Could you check a few things on this model? Use its own coordinates, in mm. Face numbers are marked on the shaded views. A direction names the side the tool comes from. Give positions to 0.01 mm unless a question says otherwise; leave off trailing zeros. Order: outer loops, then holes, each group sorted by start corner. A loop starts at its lowest first (then second) coordinate and runs counter-clockwise, first axis right, second up. Notation, with made-up numbers: (79.25, -35) -> (137.25, -35) arc R26 cw to (137.25, 0) -> close; hole circle Ø3 at (-10, -40). An arc over 180 degrees is marked (long way). One line per item, written item: value.
```python
from build123d import *
from build123d.topology import SkipClean

# Parameters (mm, degrees)
BOSS_EXTRUDE1_DEPTH          = 13.3
CHAMFER1_SIZE                = 2
CIRPATTERN1_COUNT            = 6
CHAMFER1_OF_CIRPATTERN1_SIZE = 2
CHAMFER2_SIZE                = 2
FILLET1_R                    = 1


with BuildPart() as part:
    # Sketch1 → Revolve1 (revolve)
    with BuildSketch(Plane.XY, mode=Mode.PRIVATE) as revolve1_sk:
        Polygon((-16.5, 0), (-29, 0), (-29, -8), (-23.5, -8), (-23.5, -13), (-26.75, -13), (-26.75, -17), (-20.5, -17), (-20.5, -19), (-15.5, -19), (-15.5, -6.5), (-16.5, -6.5), align=None)
    revolve(revolve1_sk.sketch.rotate(Axis((0, 0, 0), (0, -1, 0)), 270), axis=Axis((0, 0, 0), (0, -1, 0)))

    # Sketch2 → Boss-Extrude1 (add)
    with SkipClean():  # the faces are left unmerged after this step: merging them gives an invalid solid
        with BuildSketch(Plane(origin=(0, 0, 0), x_dir=(1, 0, 0), z_dir=(0, 1, 0))):
            with BuildLine():
                Line((5.154427, 16.199749), (8.792846, 27.634867))
                ThreePointArc((8.792846, 27.634867), (0, 29), (-8.792846, 27.634867))
                Line((-8.792846, 27.634867), (-5.154427, 16.199749))
                ThreePointArc((-5.154427, 16.199749), (0, 17), (5.154427, 16.199749))
            make_face()
        boss_extrude1 = extrude(amount=BOSS_EXTRUDE1_DEPTH)

    # Chamfer1
    chamfer1_edges = [part.edges().sort_by_distance(p)[0] for p in [
        (6.973637, 13.3, -21.917308),
        (-6.973637, 13.3, -21.917308),
    ]]
    chamfer(chamfer1_edges, length=CHAMFER1_SIZE)

    # CirPattern1: Boss-Extrude1 ×6 about axis
    with SkipClean():  # the faces are left unmerged after this step: merging them gives an invalid solid
        cirpattern1_axis = Axis((0, 0, 0), (0, 1, 0))
        for i in range(1, CIRPATTERN1_COUNT):
            add(boss_extrude1.rotate(cirpattern1_axis, i * 360 / CIRPATTERN1_COUNT))

    # Chamfer1 of CirPattern1
    chamfer1_of_cirpattern1_edges = [part.edges().sort_by_distance(p)[0] for p in [
        (-15.494127, 13.3, -16.998),
        (-22.467764, 13.3, -4.919308),
        (-22.467764, 13.3, 4.919308),
        (-15.494127, 13.3, 16.998),
        (-6.973637, 13.3, 21.917308),
        (6.973637, 13.3, 21.917308),
        (15.494127, 13.3, 16.998),
        (22.467764, 13.3, 4.919308),
        (22.467764, 13.3, -4.919308),
        (15.494127, 13.3, -16.998),
    ]]
    chamfer(chamfer1_of_cirpattern1_edges, length=CHAMFER1_OF_CIRPATTERN1_SIZE)

    # Chamfer2
    chamfer2_edges = [part.edges().sort_by_distance(p)[0] for p in [
        (0, -17, -26.75),
        (0, -8, -29),
    ]]
    chamfer(chamfer2_edges, length=CHAMFER2_SIZE)

    # Fillet1
    fillet1_edges = [part.edges().sort_by_distance(p)[0] for p in [
        (0, -13, -23.5),
        (0, -8, -23.5),
    ]]
    fillet(fillet1_edges, radius=FILLET1_R)


solid = part.part
```
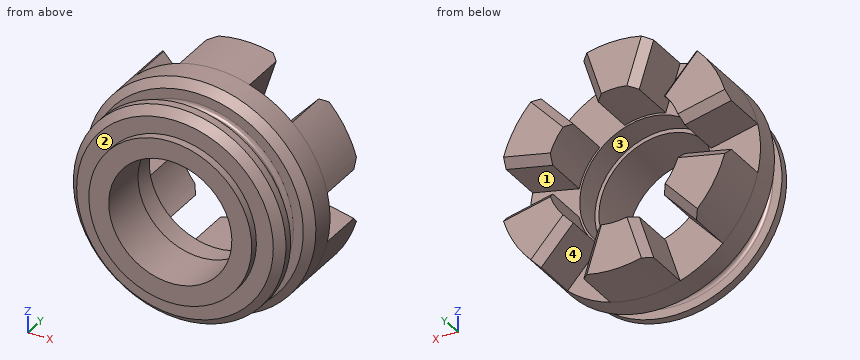
1) Suppose I cut it at C-C, the plane y = -3. Write out the boundary of the cut face in (x, z).
Answer below:
outline: circle Ø58 at (0, 0); hole circle Ø33 at (0, 0)
2) For P1, Ø12, axis at y = 4.5, z = -4.5, coming from the +X side; P2, Ø8, axis at x = 18, y = 4.5, coming from the -Z side; P3, Ø6, axis at x = -21, z = 0.5, coming from the +Y side, each with a flat end and sliding along its axis, tell me the tip position at first contact or that it passes through.
Answer below:
P1: stops at x = 29
P2: stops at z = -21.43
P3: stops at y = 0
3) Suppose I cut it at A-A, the plane y = 10. Write out the boundary of the cut face in (x, z), then the cut area to 3 significant figures.
Answer below:
outline: (-28.33, -6.2) arc R29 ccw to (-19.54, -21.43) -> (-11.45, -12.56) arc R17 cw to (-16.61, -3.64) -> close; (-28.33, 6.2) -> (-16.61, 3.64) arc R17 cw to (-11.45, 12.56) -> (-19.54, 21.43) arc R29 ccw to start; (-8.79, -27.63) arc R29 ccw to (8.79, -27.63) -> (5.15, -16.2) arc R17 cw to (-5.15, -16.2) -> close; (-8.79, 27.63) -> (-5.15, 16.2) arc R17 cw to (5.15, 16.2) -> (8.79, 27.63) arc R29 ccw to start; (11.45, -12.56) -> (19.54, -21.43) arc R29 ccw to (28.33, -6.2) -> (16.61, -3.64) arc R17 cw to start; (11.45, 12.56) arc R17 cw to (16.61, 3.64) -> (28.33, 6.2) arc R29 ccw to (19.54, 21.43) -> close
area: 1,020 mm2
4) For the marked faces 1, 2, 3 and 4, which set-ups out of +Z, -Z, +X, -X, +Y, -Y let a thin tool reach every point of the face, with its end or its side?
Answer below:
face 1: +X, +Y
face 2: -Y
face 3: +Y
face 4: -Z, +Y
5) If I drill on line 1 along X through (y, z) = (-4, 0); line 2 along X through (y, z) = (-12, 0); line 3 along Y through (x, z) = (20, -8), over which ranges is the centre line in solid material (lowest first)?
Answer below:
line 1: x = -29 to -16.5, 16.5 to 29
line 2: x = -23.5 to -15.5, 15.5 to 23.5
line 3: y = -17 to 13.3
